Print and shaded views of the part. All mm, measured from the part's lowest x, y and z. A direction names the side the tool comes from. Round coordinates to 2 decimals unless told otherwise and drop trailing zeros. Order: outer loops, then holes, each group sorted by start corner. A loop starts at its lowest first (then second) coordinate and runs counter-clockwise, first axis right, second up.
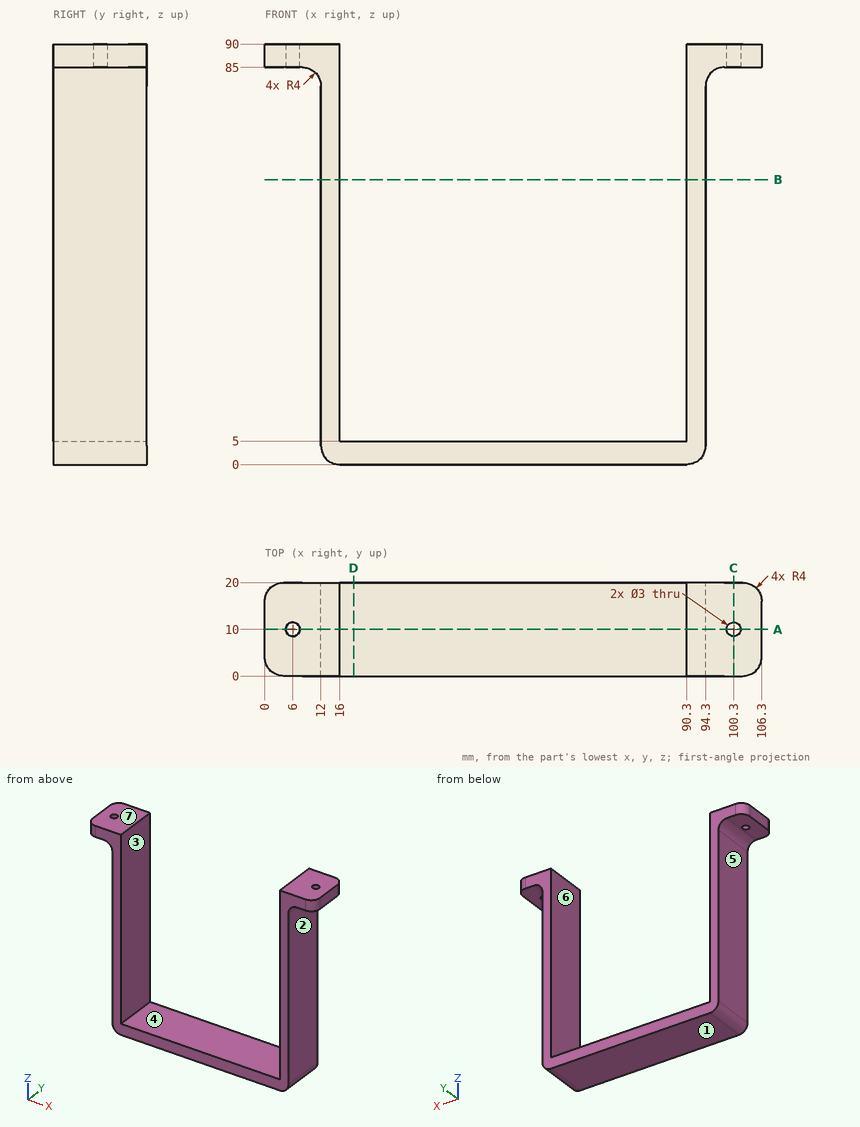
1. Cut at D-D, the plane x = 19. Write the cut outline in (y, z).
2. Cut at B-B, the plane z = 61. Write the cut outline in (x, y).
3. Tool access for the marked faces 5, 6 and 7: list every direction of +Z, -Z, +X, -X, +Y, -Y with a clear straight run to the whole face (end or side of a thin tool).
4. Cut at C-C, the plane x = 100.3. Write the cut outline in (y, z).
5. Pin check, flat tips, straight feed: P1, Ø10, axis at y = 8, z = 59, coming from the +X side; P2, Ø6, axis at y = 6, z = 52.5, coming from the -X side; P3, Ø2.5, axis at x = 2.5, y = 6.5, coming from the -Z side. Stop position of each tip, or through.
6. Mould opens along X. For the marked faces 1, 2, 3 and 4 say: released by +X, released by -X, zero draft, split by the parting line, or undercut.
7. Cut at A-A, the plane y = 10. Write the cut outline in (x, z).
8. Drill centre lines: line 1 (X direction, y = 17.75, z = 46); line 2 (Y direction, x = 6, z = 86); line 3 (Z direction, x = 42.5, y = 14.75). Where is each one in solid material? Low to high.
Outcome:
1. outline: (0, 0) - (20, 0) - (20, 5) - (0, 5) - close
2. outline: (12, 0) - (16, 0) - (16, 20) - (12, 20) - close; (90.3, 0) - (94.3, 0) - (94.3, 20) - (90.3, 20) - close
3. face 5: -Z, -X, +Y, -Y
3. face 6: +Z, +Y, -Y
3. face 7: +Z, +X, -X, +Y, -Y
4. outline: (0, 85) - (8.5, 85) - (8.5, 90) - (0, 90) - close; (11.5, 85) - (20, 85) - (20, 90) - (11.5, 90) - close
5. P1: stops at x = 94.3
5. P2: stops at x = 12
5. P3: stops at z = 85
6. face 1: zero draft
6. face 2: released by +X
6. face 3: undercut
6. face 4: undercut
7. outline: (0, 85) - (4.5, 85) - (4.5, 90) - (0, 90) - close; (7.5, 85) - (8, 85) arc R4 cw to (12, 81) - (12, 4) arc R4 ccw to (16, 0) - (90.3, 0) arc R4 ccw to (94.3, 4) - (94.3, 81) arc R4 cw to (98.3, 85) - (98.8, 85) - (98.8, 90) - (90.3, 90) - (90.3, 5) - (16, 5) - (16, 90) - (7.5, 90) - close; (101.8, 85) - (106.3, 85) - (106.3, 90) - (101.8, 90) - close
8. line 1: x = 12 to 16, 90.3 to 94.3
8. line 2: y = 0 to 8.5, 11.5 to 20
8. line 3: z = 0 to 5
